Build history of the part. All positions in model axes, mm. A direction names the side the tool comes from. Round coordinates to 2 decimals unless told otherwise and drop trailing zeros. Write each loop counter-clockwise with the first axis right and the second up, starting at its lowest first coordinate (ties: lowest second). Pieces come first, ordered by that corner, then holes. Notation, with made-up numbers: M 3.5,82.5 L 36.5,82.5 A27 cw 36.5,115.5 Z; hole C -22,58.5 d7. An arc over 180 degrees is marked long. Write item = value, one per line. Start each with the question number.
Q1. Band-saw the part on B-B on z = 44. Write the cut outline in (x, y).
Q2. Band-saw the part on D-D on y = 5. Write the cut outline in (x, z).
Q3. Drop flat-ended pins along their axis: P1, Ø9, axis at y = 20, z = -61, coming from the -X side; P2, Ø20, axis at x = 1.5, y = 14, coming from the +Z side; P3, Ø12, axis at x = 7.5, y = 18.5, coming from the -Z side. Give the stop position or say it passes through.
Q4. Pull direction X, two halves, no side cores. Call faces 1 (the flat face through (32.5, 20, -1)), 2 (the flat face through (-22.5, 20, -55)), 3 (the cylindrical face through (-27.43, 15.12, -59.92)): released by +X, released by -X, zero draft, split by the parting line, or undercut.
Q5. Band-saw the part on C-C on z = 61. Write the cut outline in (x, y).
Q6. Band-saw the part on A-A on y = 20. Write the cut outline in (x, z).
Q7. Probe L1, parallel to X at y = 37, z = -43; L2, parallel to Y at x = 26.5, z = -61; L3, parallel to Z at x = 3, y = 30. List the from-to ranges inside material, lowest first.
Q8. Tool access for faces 4 (the flat face through (-22.5, 20, 55)), 5 (the flat face through (22.5, 20, -55)), 6 (the cylindrical face through (27.57, 15.12, 62.08)): list every direction of +Z, -Z, +X, -X, +Y, -Y with a clear straight run to the whole face (end or side of a thin tool).
```python
from build123d import *

# Parameters (mm, degrees)
BOSS_EXTRUDE1_DEPTH = 40
CUT_EXTRUDE1_REACH  = 105.562
SKETCH3_R           = 5


with BuildPart() as part:
    # Sketch2 → Boss-Extrude1 (new body)
    with BuildSketch(Plane(origin=(0, 0, 0), x_dir=(1, 0, 0), z_dir=(0, 1, 0))):
        Polygon((-22.5, 70), (-22.5, 40), (22.5, 40), (22.5, 70), (32.5, 70), (32.5, -70), (22.5, -70), (22.5, -40), (-22.5, -40), (-22.5, -70), (-32.5, -70), (-32.5, 70), align=None)
    extrude(amount=BOSS_EXTRUDE1_DEPTH)

    # Cut-Extrude1: up to this face of the body (flat: up to its plane)
    cut_extrude1_end = Plane(part.part.faces().sort_by_distance((-32.5, 20, 0))[0])
    # Sketch3 → Cut-Extrude1 (cut, up to the picked face)
    with BuildSketch(Plane(origin=(32.5, 0, 0), x_dir=(0, 0, -1), z_dir=(1, 0, 0)), mode=Mode.PRIVATE) as cut_extrude1_sk1:
        with Locations((-61, 20)):
            Circle(SKETCH3_R)
    cut_extrude1_tool1 = split(extrude(cut_extrude1_sk1.sketch, amount=-CUT_EXTRUDE1_REACH, mode=Mode.PRIVATE), bisect_by=cut_extrude1_end, keep=Keep.BOTH, mode=Mode.PRIVATE)
    # Sketch3 → Cut-Extrude1 (cut, up to the picked face)
    with BuildSketch(Plane(origin=(32.5, 0, 0), x_dir=(0, 0, -1), z_dir=(1, 0, 0)), mode=Mode.PRIVATE) as cut_extrude1_sk2:
        with Locations((61, 20)):
            Circle(SKETCH3_R)
    cut_extrude1_tool2 = split(extrude(cut_extrude1_sk2.sketch, amount=-CUT_EXTRUDE1_REACH, mode=Mode.PRIVATE), bisect_by=cut_extrude1_end, keep=Keep.BOTH, mode=Mode.PRIVATE)
    add(cut_extrude1_tool1.solids().sort_by(Axis((32.5, 20, 61), (-1, 0, 0)))[0], mode=Mode.SUBTRACT)
    add(cut_extrude1_tool2.solids().sort_by(Axis((32.5, 20, -61), (-1, 0, 0)))[0], mode=Mode.SUBTRACT)


solid = part.part
```
Conclusion:
q1.outline = M -32.5,0 L -22.5,0 L -22.5,40 L -32.5,40 Z; M 22.5,0 L 32.5,0 L 32.5,40 L 22.5,40 Z
q2.outline = M -32.5,-70 L -22.5,-70 L -22.5,-40 L 22.5,-40 L 22.5,-70 L 32.5,-70 L 32.5,70 L 22.5,70 L 22.5,40 L -22.5,40 L -22.5,70 L -32.5,70 Z
q3.P1 = through
q3.P2 = 40
q3.P3 = -40
q4.face_1 = released by +X
q4.face_2 = undercut
q4.face_3 = zero draft
q5.outline = M -32.5,0 L -22.5,0 L -22.5,15 L -32.5,15 Z; M -32.5,25 L -22.5,25 L -22.5,40 L -32.5,40 Z; M 22.5,0 L 32.5,0 L 32.5,15 L 22.5,15 Z; M 22.5,25 L 32.5,25 L 32.5,40 L 22.5,40 Z
q6.outline = M -32.5,-70 L -22.5,-70 L -22.5,-66 L -32.5,-66 Z; M -32.5,-56 L -22.5,-56 L -22.5,-40 L 22.5,-40 L 22.5,-56 L 32.5,-56 L 32.5,56 L 22.5,56 L 22.5,40 L -22.5,40 L -22.5,56 L -32.5,56 Z; M -32.5,66 L -22.5,66 L -22.5,70 L -32.5,70 Z; M 22.5,-70 L 32.5,-70 L 32.5,-66 L 22.5,-66 Z; M 22.5,66 L 32.5,66 L 32.5,70 L 22.5,70 Z
q7.L1 = -32.5 to -22.5, 22.5 to 32.5
q7.L2 = 0 to 15, 25 to 40
q7.L3 = -40 to 40
q8.face_4 = +Z, +Y, -Y
q8.face_5 = -Z, +Y, -Y
q8.face_6 = +X, -X
